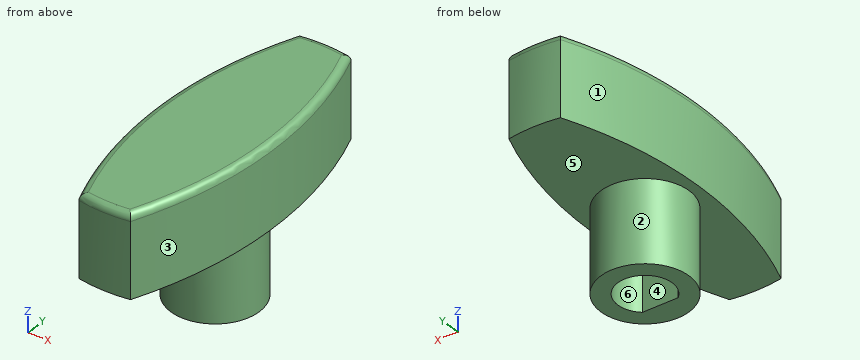
from build123d import *

# Parameters (mm, degrees)
SKETCH1_R           = 6.5
BOSS_EXTRUDE1_DEPTH = 12
BOSS_EXTRUDE2_DEPTH = 12
FILLET1_R           = 1


with BuildPart() as part:
    # Sketch1 → Boss-Extrude1 (new body)
    with BuildSketch(Plane.XY):
        Circle(SKETCH1_R)
        with BuildLine():
            Line((-2.645751311, -3), (2.645751311, -3))
            ThreePointArc((2.645751311, -3), (0, 4), (-2.645751311, -3))
        make_face(mode=Mode.SUBTRACT)
    extrude(amount=BOSS_EXTRUDE1_DEPTH)

    # Sketch2 → Boss-Extrude2 (add)
    with BuildSketch(Plane.XY.offset(12)):
        with BuildLine():
            ThreePointArc((3.8, 21.669333169), (8, 0), (3.8, -21.669333169))
            ThreePointArc((3.8, -21.669333169), (0, -22), (-3.8, -21.669333169))
            ThreePointArc((-3.8, -21.669333169), (-8, 0), (-3.8, 21.669333169))
            ThreePointArc((-3.8, 21.669333169), (0, 22), (3.8, 21.669333169))
        make_face()
    extrude(amount=BOSS_EXTRUDE2_DEPTH)

    # Fillet1
    fillet1_edges = [part.edges().sort_by_distance(p)[0] for p in [
        (0, 22, 24),
        (-8, 0, 24),
        (0, -22, 24),
        (8, 0, 24),
    ]]
    fillet(fillet1_edges, radius=FILLET1_R)


solid = part.part
Could you check a few things on this model? Use its own coordinates, in mm. Face numbers are marked on the shaded views. A direction names the side the tool comes from. Round coordinates to 2 decimals unless told otherwise and drop trailing zeros. Order: outer loops, then holes, each group sorted by start corner. A loop starts at its lowest first (then second) coordinate and runs counter-clockwise, first axis right, second up.
(1) I'm going to push flat-ended pins straight in: pin 1 (5.5 mm diameter, centred on x = -1.5, y = 0.5, fed in from -Z); pin 2 (1.5 mm diameter, centred on x = 6, z = 8.5, fed in from -Y); pin 3 (5 mm diameter, centred on x = -1, y = 9, fed in from -Z); pin 4 (4 mm diameter, centred on y = -2.5, z = 11, fed in from -X). Where does each tip first touch, or does it pass through?
Response values:
pin 1: stops at z = 0
pin 2: stops at y = -3.83
pin 3: stops at z = 12
pin 4: stops at x = -7.99
(2) Imagine slicing it at C-C (z = 10). Write out the boundary of the cut face in (x, y), plus the area to 3 significant figures.
Response values:
outline: circle Ø13 at (0, 0); hole (-2.65, -3) - (2.65, -3) arc R4 ccw (long way) to start
area: 86.1 mm2
(3) Which directions (+Z, -Z, +X, -X, +Y, -Y) give clear straight access to the entire face, cutting with the end or side of a thin tool? Please do the marked faces 1 and 2.
Response values:
face 1: +Z, -Z, -X
face 2: -Z
(4) Please list where these lines run through material, in increasing order: line 1 along Z through (x, y) = (-1.75, -18); line 2 along X through (y, z) = (15.5, 19.5); line 3 along X through (y, z) = (1, 2.5).
Response values:
line 1: z = 12 to 24
line 2: x = -5.89 to 5.89
line 3: x = -6.42 to -3.87, 3.87 to 6.42
(5) Imagine slicing it at D-D (z = 13). Write out the boundary of the cut face in (x, y), plus the area to 3 significant figures.
Response values:
outline: (-3.8, -21.67) arc R22 ccw to (3.8, -21.67) arc R58 ccw to (3.8, 21.67) arc R22 ccw to (-3.8, 21.67) arc R58 ccw to start
area: 577 mm2
(6) Imagine slicing it at B-B (y = 0). Write out the boundary of the cut face in (x, z), plus the area to 3 significant figures.
Response values:
outline: (-8, 12) - (-6.5, 12) - (-6.5, 0) - (-4, 0) - (-4, 12) - (4, 12) - (4, 0) - (6.5, 0) - (6.5, 12) - (8, 12) - (8, 23) arc R1 ccw to (7, 24) - (-7, 24) arc R1 ccw to (-8, 23) - close
area: 252 mm2
(7) Imagine slicing it at A-A (x = 0). Write out the boundary of the cut face in (y, z).
Response values:
outline: (-22, 12) - (-6.5, 12) - (-6.5, 0) - (-3, 0) - (-3, 12) - (4, 12) - (4, 0) - (6.5, 0) - (6.5, 12) - (22, 12) - (22, 23) arc R1 ccw to (21, 24) - (-21, 24) arc R1 ccw to (-22, 23) - close
(8) If we mould it in two halves opening along Y, with no side actions, what happens to the marked faces 3, 4, 5 and 6? For each: released by +Y, released by -Y, zero draft, split by the parting line, or undercut.
Response values:
face 3: split by the parting line
face 4: undercut
face 5: zero draft
face 6: undercut
